The figure shows three views and two pictorial views of one solid part (mm, origin at its lowest corner). Answer the questions. A direction names the side the tool comes from. Coordinates: 2 decimals unless noted, no trailing zeros. Loops run counter-clockwise (first coordinate to the right, second up) from the corner with the lowest first, then second, coordinate; pieces in that order, holes last.
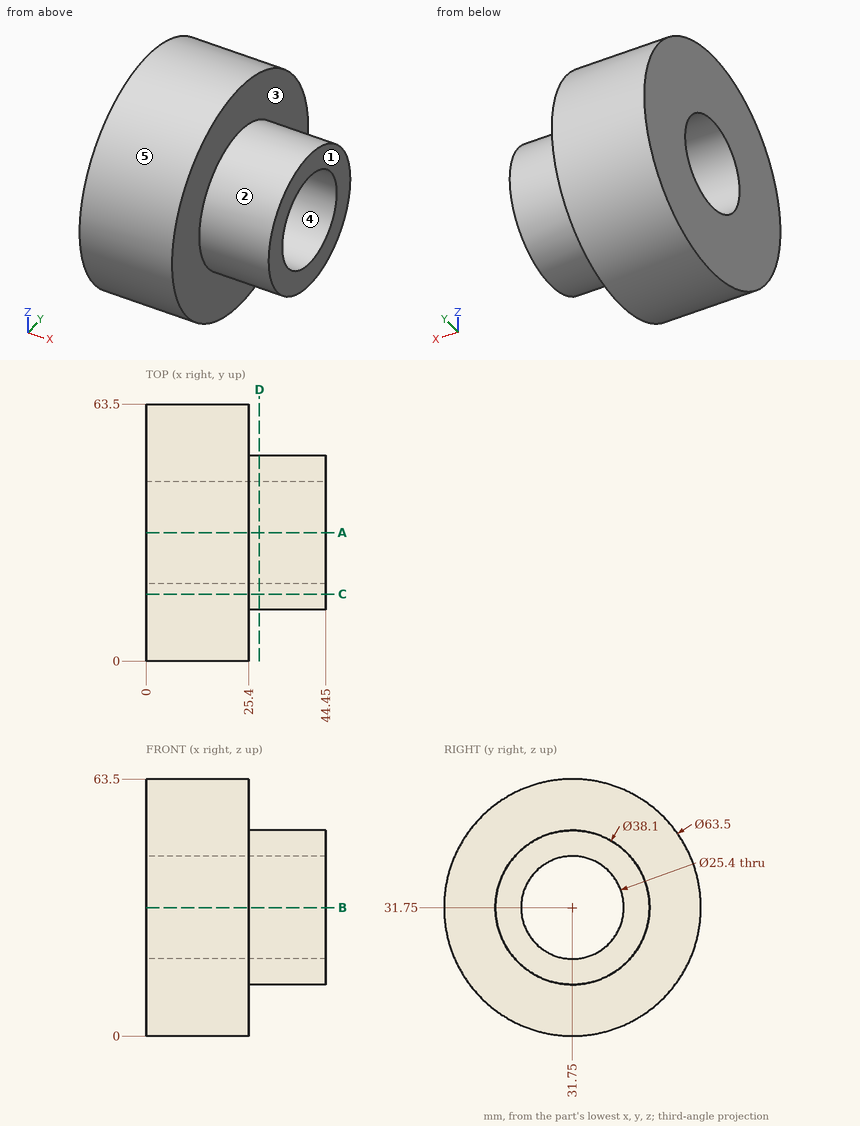
Q1. A cutting plane is placed at C-C (y = 16.5). Give the vertices of the cut face in (x, z), then the cut area to 3 significant figures.
Findings below:
outline: (0, 3.9) - (25.4, 3.9) - (25.4, 20.33) - (44.45, 20.33) - (44.45, 43.17) - (25.4, 43.17) - (25.4, 59.6) - (0, 59.6) - close
area: 1,850 mm2
Q2. Straight lines are drawn through the part: probe 1 along Z at (x, y) = (36.5, 31.75); probe 2 along Z at (x, y) = (22.5, 31.75); probe 3 along X at (y, z) = (31, 7.5). For each, find the intervals that lie inside material, in ascending order.
Findings below:
probe 1: z = 12.7 to 19.05, 44.45 to 50.8
probe 2: z = 0 to 19.05, 44.45 to 63.5
probe 3: x = 0 to 25.4
Q3. Determine the mould class of the marked faces 3, 4 and 5 for opening direction Z: +Z half, -Z half, draft (parallel to the pull), parting line (faces both ways), or undercut.
Findings below:
face 3: draft
face 4: undercut
face 5: parting line
Q4. Flat-ended cylindrical pins translate along their axes: pin 1 Ø8 at (x, y) = (10.5, 12.5) entering from -Z; pin 2 Ø1 at (x, z) = (20, 9.5) entering from -Y; pin 3 Ø1.5 at (y, z) = (27, 52) entering from -X; pin 4 Ø5 at (x, z) = (9.5, 11) entering from +Y. Find the tip coordinate at first contact, or state that the pin passes through.
Findings below:
pin 1: stops at z = 3.9
pin 2: stops at y = 8.62
pin 3: stops at x = 0
pin 4: stops at y = 57.73
Q5. Which of the six approach directions +Z, -Z, +X, -X, +Y, -Y give full straight-line access (tool end or side, diameter ignored) to the marked faces 1 and 2?
Findings below:
face 1: +Z, -Z, +X, +Y, -Y
face 2: +X
Q6. A cutting plane is placed at A-A (y = 31.75). Give the vertices of the cut face in (x, z), then the cut area to 3 significant figures.
Findings below:
outline: (0, 0) - (25.4, 0) - (25.4, 12.7) - (44.45, 12.7) - (44.45, 19.05) - (0, 19.05) - close; (0, 44.45) - (44.45, 44.45) - (44.45, 50.8) - (25.4, 50.8) - (25.4, 63.5) - (0, 63.5) - close
area: 1,210 mm2
Q7. A cutting plane is placed at D-D (x = 28). Give the vertices of the cut face in (y, z), then the cut area to 3 significant figures.
Findings below:
outline: circle Ø38.1 at (31.75, 31.75); hole circle Ø25.4 at (31.75, 31.75)
area: 633 mm2
